Design review of the part built by this model. Coordinates are the model's own, in mm. Face numbers are marked on the shaded views. A direction names the side the tool comes from. Coordinates: 2 decimals unless noted, no trailing zeros. Write each loop counter-clockwise with the first axis right and the second up, starting at its lowest first coordinate (ties: lowest second). Pieces come first, ordered by that corner, then holes. Notation, with made-up numbers: (-22.75, 41) -> (35.25, 41) arc R7 ccw to (35.25, 51) -> close; hole circle Ø10 at (18, 74.25). An arc over 180 degrees is marked (long way). Return JSON: item names as keys, results as strings. Group by question number.
from build123d import *

# Parameters (mm, degrees)
SKETCH1_W           = 82
SKETCH1_H           = 25
BOSS_EXTRUDE1_DEPTH = 14.2
CUT_EXTRUDE3_DEPTH  = 14.2
BOSS_EXTRUDE2_DEPTH = 1
BOSS_EXTRUDE3_START = -13.2
BOSS_EXTRUDE3_DEPTH = 1
CUT_EXTRUDE4_START  = -6.45
CUT_EXTRUDE4_DEPTH  = 3.25
CUT_EXTRUDE5_DEPTH  = 4.5
CUT_EXTRUDE6_DEPTH  = 14.2
SKETCH8_R           = 1.625
CUT_EXTRUDE7_DEPTH  = 5
SKETCH10_W          = 25
SKETCH10_H          = 10.138458538
BOSS_EXTRUDE4_DEPTH = 9.9
SKETCH11_R          = 9.75
CUT_EXTRUDE8_DEPTH  = 4
SKETCH12_R          = 1.625
CUT_EXTRUDE9_DEPTH  = 5.9
CIRPATTERN1_COUNT   = 3
SKETCH13_R          = 2.625
CUT_EXTRUDE10_DEPTH = 5.9


with BuildPart() as part:
    # Sketch1 → Boss-Extrude1 (new body)
    with BuildSketch(Plane.XY):
        with Locations((0, 12.5)):
            Rectangle(SKETCH1_W, SKETCH1_H)
    extrude(amount=BOSS_EXTRUDE1_DEPTH)

    # Sketch2 → Cut-Extrude3 (cut)
    with BuildSketch(Plane(origin=(0, 0, 0), x_dir=(-1, 0, 0), z_dir=(0, 0, -1))):
        with BuildLine():
            Line((-31, 0), (-19, 0))
            ThreePointArc((-19, 0), (-25, 6), (-31, 0))
        make_face()
        with BuildLine():
            Line((19, 0), (31, 0))
            ThreePointArc((31, 0), (25, 6), (19, 0))
        make_face()
    extrude(amount=-CUT_EXTRUDE3_DEPTH, mode=Mode.SUBTRACT)

    # Sketch4 → Boss-Extrude2 (add)
    with BuildSketch(Plane(origin=(0, 0, 0), x_dir=(-1, 0, 0), z_dir=(0, 0, -1))):
        with BuildLine():
            Line((-30.75, 0), (-31, 0))
            ThreePointArc((-31, 0), (-25, 6), (-19, 0))
            Line((-19, 0), (-19.25, 0))
            ThreePointArc((-19.25, 0), (-25, 5.75), (-30.75, 0))
        make_face()
        with BuildLine():
            Line((19, 0), (19.25, 0))
            ThreePointArc((19.25, 0), (25, 5.75), (30.75, 0))
            Line((30.75, 0), (31, 0))
            ThreePointArc((31, 0), (25, 6), (19, 0))
        make_face()
    extrude(amount=-BOSS_EXTRUDE2_DEPTH)

    # Sketch4<2> → Boss-Extrude3 (add)
    with BuildSketch(Plane(origin=(0, 0, 0), x_dir=(-1, 0, 0), z_dir=(0, 0, -1)).offset(BOSS_EXTRUDE3_START)):
        with BuildLine():
            Line((-30.75, 0), (-31, 0))
            ThreePointArc((-31, 0), (-25, 6), (-19, 0))
            Line((-19, 0), (-19.25, 0))
            ThreePointArc((-19.25, 0), (-25, 5.75), (-30.75, 0))
        make_face()
        with BuildLine():
            Line((19, 0), (19.25, 0))
            ThreePointArc((19.25, 0), (25, 5.75), (30.75, 0))
            Line((30.75, 0), (31, 0))
            ThreePointArc((31, 0), (25, 6), (19, 0))
        make_face()
    extrude(amount=-BOSS_EXTRUDE3_DEPTH)

    # Sketch5 → Cut-Extrude4 (cut)
    with BuildSketch(Plane(origin=(0, 0, 0), x_dir=(-1, 0, 0), z_dir=(0, 0, -1)).offset(CUT_EXTRUDE4_START)):
        with BuildLine():
            Line((-6.5, 0), (6.5, 0))
            ThreePointArc((6.5, 0), (0, 6.5), (-6.5, 0))
        make_face()
    extrude(amount=-CUT_EXTRUDE4_DEPTH, mode=Mode.SUBTRACT)

    # Sketch6 → Cut-Extrude5 (cut)
    with BuildSketch(Plane(origin=(0, 0, 14.2), x_dir=(-1, 0, 0), z_dir=(0, 0, -1))):
        with BuildLine():
            Line((-2.625, 0), (2.625, 0))
            ThreePointArc((2.625, 0), (0, 2.625), (-2.625, 0))
        make_face()
    extrude(amount=CUT_EXTRUDE5_DEPTH, mode=Mode.SUBTRACT)

    # Sketch7 → Cut-Extrude6 (cut)
    with BuildSketch(Plane(origin=(0, 0, 0), x_dir=(-1, 0, 0), z_dir=(0, 0, -1))):
        with BuildLine():
            Line((-41, 5), (-33.5, 5))
            ThreePointArc((-33.5, 5), (-29.896033736, 8.560306867), (-25, 9.861541462))
            Line((-25, 9.861541462), (25, 9.861541462))
            ThreePointArc((25, 9.861541462), (29.896033736, 8.560306867), (33.5, 5))
            Line((33.5, 5), (41, 5))
            Line((41, 5), (41, 25))
            Line((41, 25), (-41, 25))
            Line((-41, 25), (-41, 5))
        make_face()
    extrude(amount=-CUT_EXTRUDE6_DEPTH, mode=Mode.SUBTRACT)

    # Sketch8 → Cut-Extrude7 (cut)
    with BuildSketch(Plane(origin=(0, 5, 0), x_dir=(1, 0, 0), z_dir=(0, 1, 0))):
        with Locations(Location((37.25, -3.75, 0), (0, 0, 270))):
            Circle(SKETCH8_R)
        with Locations(Location((37.25, -10.45, 0), (0, 0, 270))):
            Circle(SKETCH8_R)
        with Locations(Location((-37.25, -3.75, 0), (0, 0, 270))):
            Circle(SKETCH8_R)
        with Locations(Location((-37.25, -10.45, 0), (0, 0, 270))):
            Circle(SKETCH8_R)
    extrude(amount=-CUT_EXTRUDE7_DEPTH, mode=Mode.SUBTRACT)

    # Sketch10 → Boss-Extrude4 (add)
    with BuildSketch(Plane.XY.offset(14.2)):
        with Locations((0, 14.930770731)):
            Rectangle(SKETCH10_W, SKETCH10_H)
        with BuildLine():
            Line((-12.5, 20), (12.5, 20))
            ThreePointArc((12.5, 20), (0, 32.5), (-12.5, 20))
        make_face()
    extrude(amount=-BOSS_EXTRUDE4_DEPTH)

    # Sketch11 → Cut-Extrude8 (cut)
    with BuildSketch(Plane(origin=(0, 0, 4.3), x_dir=(-1, 0, 0), z_dir=(0, 0, -1))):
        with Locations((0, 20)):
            Circle(SKETCH11_R)
    extrude(amount=-CUT_EXTRUDE8_DEPTH, mode=Mode.SUBTRACT)

    # Sketch12 → Cut-Extrude9 (cut)
    with BuildSketch(Plane(origin=(0, 0, 8.3), x_dir=(-1, 0, 0), z_dir=(0, 0, -1))):
        with Locations((0, 26.35)):
            Circle(SKETCH12_R)
    cut_extrude9 = extrude(amount=-CUT_EXTRUDE9_DEPTH, mode=Mode.SUBTRACT)

    # CirPattern1: Cut-Extrude9 ×3 about axis
    cirpattern1_axis = Axis((0, 20, 0), (0, 0, 1))
    for i in range(1, CIRPATTERN1_COUNT):
        add(cut_extrude9.rotate(cirpattern1_axis, i * 360 / CIRPATTERN1_COUNT), mode=Mode.SUBTRACT)

    # Sketch13 → Cut-Extrude10 (cut)
    with BuildSketch(Plane(origin=(0, 0, 8.3), x_dir=(-1, 0, 0), z_dir=(0, 0, -1))):
        with Locations((0, 20)):
            Circle(SKETCH13_R)
    extrude(amount=-CUT_EXTRUDE10_DEPTH, mode=Mode.SUBTRACT)


solid = part.part
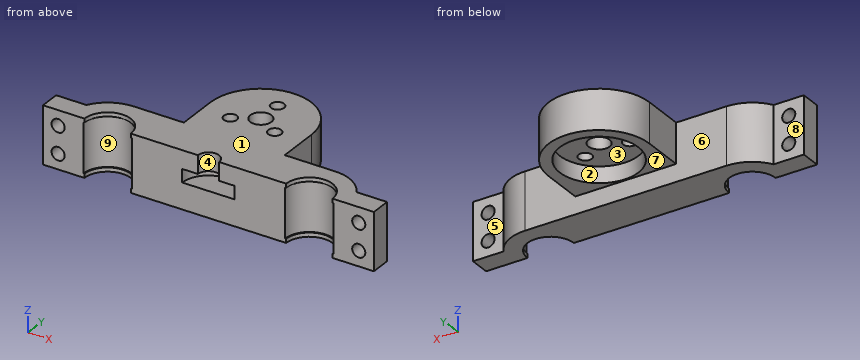
Q1. We need section C-C on x = 0. Write out the cut boundary in (y, z) (3 decimals), plus the area to 3 significant figures.
Q2. We need section B-B on y = 26.35. Write out the cut boundary in (x, z) (3 decimals).
Q3. For the marked faces 5, 6, 7, 8 and 9, list the 3-axis set-ups (+Z, -Z, +X, -X, +Y, -Y) from which the entire face can be reached by the end or side of a thin tool; tool diameter is ignored.
Q4. Wall thickness on L1, parallel to Y at x = 0, z = 11.7 (3 decimals); L2, parallel to X at y = 16.5, z = 13.25; L3, parallel to Y at x = 0, z = 9.6 (3 decimals): over which ranges is each line inside the solid? List them lowest first.
Q5. We need section A-A on x = 37.25. Write out the cut boundary in (y, z) (3 decimals), plus the area to 3 significant figures.
Q6. We need section D-D on x = 20. Write out the cut boundary in (y, z), plus the area to 3 significant figures.
Q7. The part is to be moulded in two halves that separate along Y. For the marked faces 1, 2, 3 and 4, say which applies: +Y half, -Y half, draft (parallel to the pull), parting line (faces both ways), or undercut.
Q8. For P1, Ø7, axis at x = 3, z = 10, coming from the +Y side; P2, Ø4, axis at x = 37.25, z = 3.75, coming from the +Y side; P3, Ø6, axis at y = 24, z = 4, coming from the -X side; P4, Ø8.5, axis at x = 0, y = 20, coming from the -Z side, all flat-tipped, find the tip position at first contact; note any pin that passes through.
Findings below:
{
 "1": {"outline": "(0, 0) -> (9.862, 0) -> (9.862, 4.3) -> (10.25, 4.3) -> (10.25, 8.3) -> (17.375, 8.3) -> (17.375, 14.2) -> (2.625, 14.2) -> (2.625, 9.7) -> (6.5, 9.7) -> (6.5, 6.45) -> (0, 6.45) -> close; (22.625, 8.3) -> (24.725, 8.3) -> (24.725, 14.2) -> (22.625, 14.2) -> close; (27.975, 8.3) -> (29.75, 8.3) -> (29.75, 4.3) -> (32.5, 4.3) -> (32.5, 14.2) -> (27.975, 14.2) -> close", "area": "203 mm^2"},
 "2": {"outline": "(-10.767, 4.3) -> (-7.399, 4.3) -> (-7.399, 8.3) -> (-1.625, 8.3) -> (-1.625, 14.2) -> (-10.767, 14.2) -> close; (1.625, 8.3) -> (7.399, 8.3) -> (7.399, 4.3) -> (10.767, 4.3) -> (10.767, 14.2) -> (1.625, 14.2) -> close"},
 "3": {"face 5": "+Z, -Z, +X, +Y", "face 6": "-Z, +Y", "face 7": "-Z, +X, -X, +Y", "face 8": "+Z, -Z, -X, +Y", "face 9": "-Y"},
 "4": {"L1": "y = 2.625 to 17.375, 22.625 to 24.725, 27.975 to 32.5", "L2": "x = -12.5 to -7.09, -3.91 to 3.91, 7.09 to 12.5", "L3": "y = 6.5 to 17.375, 22.625 to 24.725, 27.975 to 32.5"},
 "5": {"outline": "(0, 0) -> (5, 0) -> (5, 2.125) -> (0, 2.125) -> close; (0, 5.375) -> (5, 5.375) -> (5, 8.825) -> (0, 8.825) -> close; (0, 12.075) -> (5, 12.075) -> (5, 14.2) -> (0, 14.2) -> close", "area": "38.5 mm^2"},
 "6": {"outline": "(2.84, 0) -> (9.86, 0) -> (9.86, 14.2) -> (2.84, 14.2) -> (2.84, 13.2) -> (3.32, 13.2) -> (3.32, 1) -> (2.84, 1) -> close", "area": "93.9 mm^2"},
 "7": {"face 1": "draft", "face 2": "undercut", "face 3": "undercut", "face 4": "-Y half"},
 "8": {"P1": "stops at y = 32.5", "P2": "stops at y = 5", "P3": "stops at x = -12.46", "P4": "stops at z = 8.3"}
}
